Read the model definition and answer for the solid it produces. Units are mm, in the model's axes. Face numbers are marked on the shaded views. A direction names the side the tool comes from. Give positions to 0.01 mm unless a question says otherwise; leave off trailing zeros. Loops run counter-clockwise (first coordinate to the right, second up) from the corner with the lowest first, then second, coordinate; pieces in that order, holes last. Notation, with made-up numbers: (62.25, -26) - (113.25, -26) arc R20 cw to (113.25, 4) - close; hole circle Ø3 at (1.25, 67.25). An arc over 180 degrees is marked (long way). Write item = value, one per line.
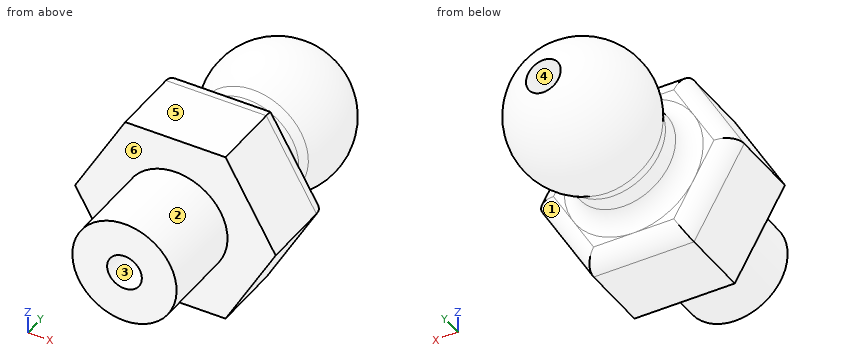
```python
from build123d import *

# Parameters (mm, degrees)
SKETCH2_R          = 10.06808877
CUT_EXTRUDE1_DEPTH = 10
FILLET1_R          = 1
FILLET2_R          = 1
SKETCH3_W          = 1
SKETCH3_H          = 0.936459383
CUT_EXTRUDE2_DEPTH = 3
CIRPATTERN1_COUNT  = 6


with BuildPart() as part:
    # Sketch1 → Revolve1 (revolve)
    with BuildSketch(Plane.XY, mode=Mode.PRIVATE) as revolve1_sk:
        with BuildLine():
            Line((-1, 0), (-3, 0))
            Line((-3, 0), (-3, 5))
            Line((-3, 5), (-6, 5))
            Line((-6, 5), (-6, 10))
            Line((-6, 10), (-3, 10))
            Line((-3, 10), (-3, 12.354248689))
            ThreePointArc((-3, 12.354248689), (-3.824065295, 16.173253859), (-1, 18.872983346))
            Line((-1, 18.872983346), (-1, 16.732050808))
            ThreePointArc((-1, 16.732050808), (-1.732050808, 16), (-2, 15))
            Line((-2, 15), (-2, 7))
            Line((-2, 7), (-1, 7))
            Line((-1, 7), (-1, 0))
        make_face()
    revolve(revolve1_sk.sketch.rotate(Axis((0, 0, 0), (0, 1, 0)), 270), axis=Axis((0, 0, 0), (0, 1, 0)))

    # Sketch2 → Cut-Extrude1 (cut)
    with BuildSketch(Plane(origin=(0, 10, 0), x_dir=(1, 0, 0), z_dir=(0, 1, 0))):
        Circle(SKETCH2_R)
        Polygon((5.773502692, 0), (2.886751346, 5), (-2.886751346, 5), (-5.773502692, 0), (-2.886751346, -5), (2.886751346, -5), align=None, mode=Mode.SUBTRACT)
    extrude(amount=-CUT_EXTRUDE1_DEPTH, mode=Mode.SUBTRACT)

    # Fillet1
    fillet1_edges = [part.edges().sort_by_distance(p)[0] for p in [
        (0, 12.354248689, 3),
        (0, 10, 3),
    ]]
    fillet(fillet1_edges, radius=FILLET1_R)

    # Fillet2
    fillet2_edges = [part.edges().sort_by_distance(p)[0] for p in [
        (4.330127019, 10, 2.5),
        (0, 10, 5),
        (-4.330127019, 10, 2.5),
        (-4.330127019, 10, -2.5),
        (0, 10, -5),
        (4.330127019, 10, -2.5),
    ]]
    fillet(fillet2_edges, radius=FILLET2_R - 0.0001)  # a hair under: the kernel refuses the full size

    # Sketch3 → Cut-Extrude2 (cut)
    with BuildSketch(Plane(origin=(0, 10, 0), x_dir=(1, 0, 0), z_dir=(0, 1, 0))):
        with Locations((0, 1.831770309)):
            Rectangle(SKETCH3_W, SKETCH3_H)
    cut_extrude2 = extrude(amount=-CUT_EXTRUDE2_DEPTH, mode=Mode.SUBTRACT)

    # CirPattern1: Cut-Extrude2 ×6 about axis
    cirpattern1_axis = Axis((0, 0, 0), (0, 1, 0))
    for i in range(1, CIRPATTERN1_COUNT):
        add(cut_extrude2.rotate(cirpattern1_axis, i * 360 / CIRPATTERN1_COUNT), mode=Mode.SUBTRACT)


solid = part.part
```
1) A tool of negligible diameter and unlimited length cuts with its end or side. For the marked faces 5 and 6, from which of +Z, -Z, +X, -X, +Y, -Y can it reach the whole face along a straight path? Write none if from no direction.
Output:
face_5 = +Z, +X, -X, +Y, -Y
face_6 = -Y
2) Each of these flat-tipped pins is pushed along its axis until it touches: P1, Ø1.5, axis at x = 0, y = 14.5, coming from the -Z side; P2, Ø6, axis at y = 16.5, z = -1, coming from the +X side; P3, Ø1.2, axis at x = 0, z = 0, coming from the +Y side (1 decimal). Where does it stop, or does it pass through?
Output:
P1 = -4
P2 = 4
P3 = through
3) A cutting plane is placed at C-C on y = 15.25. Determine the outline of the cut face in (x, z).
Output:
outline = circle Ø7.98 at (0, 0); hole circle Ø3.97 at (0, 0)
4) The mould has two halves that part along X. Classify the marked faces 1, 2, 3 and 4: pulls with the +X half, pulls with the -X half, needs draft (parallel to the pull), parting line crosses it, or undercut.
Output:
face_1 = pulls with the +X half
face_2 = parting line crosses it
face_3 = undercut
face_4 = undercut
5) Find the intervals of material crossed by probe 1 along X at (y, z) = (4.5, 0); probe 2 along Z at (x, y) = (0, 9); probe 3 along Y at (x, z) = (0, 1.5), in increasing order.
Output:
probe_1 = -3 to -1, 1 to 3
probe_2 = -5 to -2.3, 2.3 to 5
probe_3 = 0 to 7, 16.32 to 18.71
6) A cutting plane is placed at B-B on y = 2.5. Determine the outline of the cut face in (x, z).
Output:
outline = circle Ø6 at (0, 0); hole circle Ø2 at (0, 0)
